```python
from build123d import *

# Parameters (mm, degrees)
SKETCH1_R           = 16.764
BOSS_EXTRUDE1_DEPTH = 63.5
SKETCH2_R           = 14.351
CUT_EXTRUDE1_DEPTH  = 166.37
CHAMFER1_SIZE       = 1.27


with BuildPart() as part:
    # Sketch1 → Boss-Extrude1 (new body)
    with BuildSketch(Plane(origin=(0, 0, 0), x_dir=(1, 0, 0), z_dir=(0, 1, 0))):
        with Locations((-13.41463778, 13.288084593)):
            Circle(SKETCH1_R)
    extrude(amount=BOSS_EXTRUDE1_DEPTH)

    # Sketch2 → Cut-Extrude1 (cut)
    with BuildSketch(Plane(origin=(0, 0, 0), x_dir=(1, 0, 0), z_dir=(0, 1, 0))):
        with Locations((-13.258576493, 13.278033005)):
            Circle(SKETCH2_R)
    extrude(amount=CUT_EXTRUDE1_DEPTH, mode=Mode.SUBTRACT)

    # Chamfer1
    chamfer1_edges = [part.edges().sort_by_distance(p)[0] for p in [
        (-30.17863778, 63.5, -13.288084593),
    ]]
    chamfer(chamfer1_edges, length=CHAMFER1_SIZE)


solid = part.part
```
Verification items for the finished model (mm, model axes). Coordinates: 2 decimals unless noted, no trailing zeros. Loops run counter-clockwise (first coordinate to the right, second up) from the corner with the lowest first, then second, coordinate; pieces in that order, holes last. Notation, with made-up numbers: (25.5, 55) -> (37.5, 55) arc R30 cw to (37.5, 82) -> close; hole circle Ø10 at (72.5, -4.5). An arc over 180 degrees is marked (long way). Answer in a Markdown table with one row per item. Add a question column.
1. Draft check along Z on faces 1 (the face through (-26, 63.5, -6)), 2 (the face through (-26.72, 30.68, -3.09)), 3 (the face through (-27.596, 31.306, -13.909)). Enter one of: +Z half, -Z half, draft (parallel to the pull), parting line (faces both ways), or undercut.
2. Material ranges on probe 1 along Z at (x, y) = (-7, 17.5); probe 2 along Z at (x, y) = (-12, 22); probe 3 along X at (y, z) = (5, 0), recorded low to high. Write a range as [from, to].
3. Section check A-A, the plane y = 22.5. Enter the section's corners in (x, z), then the cut area to 3 significant figures.
4. Depth check by flat-ended pin: P1, Ø4, axis at y = 21, z = -10, coming from the +X side; P2, Ø6, axis at x = -21.5, y = 28, coming from the -Z side; P3, Ø1, axis at y = 29.5, z = -10.5, coming from the +X side. Enter the tip coordinate at first touch or a pass-through.
Derived:
| question | item | result |
|---|---|---|
| 1 | face 1 | draft |
| 1 | face 2 | parting line |
| 1 | face 3 | undercut |
| 2 | probe 1 | z = [-28.78, -26.19], [-0.36, 2.2] |
| 2 | probe 2 | z = [-29.99, -27.57], [1.02, 3.42] |
| 2 | probe 3 | x = [-23.64, -18.7], [-7.81, -3.19] |
| 3 | outline | circle Ø33.53 at (-13.41, -13.29); hole circle Ø28.7 at (-13.26, -13.28) |
| 3 | area | 236 mm² |
| 4 | P1 | stops at x = 3.3 |
| 4 | P2 | stops at z = -29.26 |
| 4 | P3 | stops at x = 3.19 |
